Input: dimensioned drawing with shaded views. Units: mm. Origin: part minimum x, y, z. A direction names the side the tool comes from. Round coordinates to 2 decimals unless told otherwise and drop trailing zeros. Loops run counter-clockwise (first coordinate to the right, second up) from the corner with the lowest first, then second, coordinate; pieces in that order, holes last. Notation, with made-up numbers: (18.25, 78) - (59.25, 78) arc R20 ccw to (59.25, 104) - close; hole circle Ø8 at (80.5, 42). An arc over 180 degrees is marked (long way). One line per question, with ' | ' between items. Start each with the question number.
1. Cut plane A-A (x = 64.5). Return loops of the section in (y, z).
2. Pin query (flat end, axial travel): pin 1 (10 mm diameter, centred on x = 64, y = 84, fed in from +Z); pin 2 (5.5 mm diameter, centred on y = 80.5, z = 2.5, fed in from +X); pin 3 (5.5 mm diameter, centred on y = 34, z = 8.5, fed in from -X); pin 4 (4 mm diameter, centred on x = 131.5, z = 8.5, fed in from -Y). Return the tip coordinate at first contact, or that it passes through.
3. Cut plane C-C (z = 7.5). Return loops of the section in (x, y).
4. Cut plane B-B (y = 26.5). Return loops of the section in (x, z).
5. Cut plane D-D (x = 21.5). Return loops of the section in (y, z), then the cut area to 3 significant figures.
6. Ray query, line 1 (Y direction, x = 37, z = 3.5); line 2 (Z direction, x = 17, y = 57.5); line 3 (Y direction, x = 97, z = 8.5). Return the intervals inside material, ascending.
7. Access query for the marked faces 1, 2, 3 and 4. Directions: +Z, -Z, +X, -X, +Y, -Y. A direction counts if a zero-diameter tool reaches every point of the face in a straight line with its end or side. Return the directions, or none.
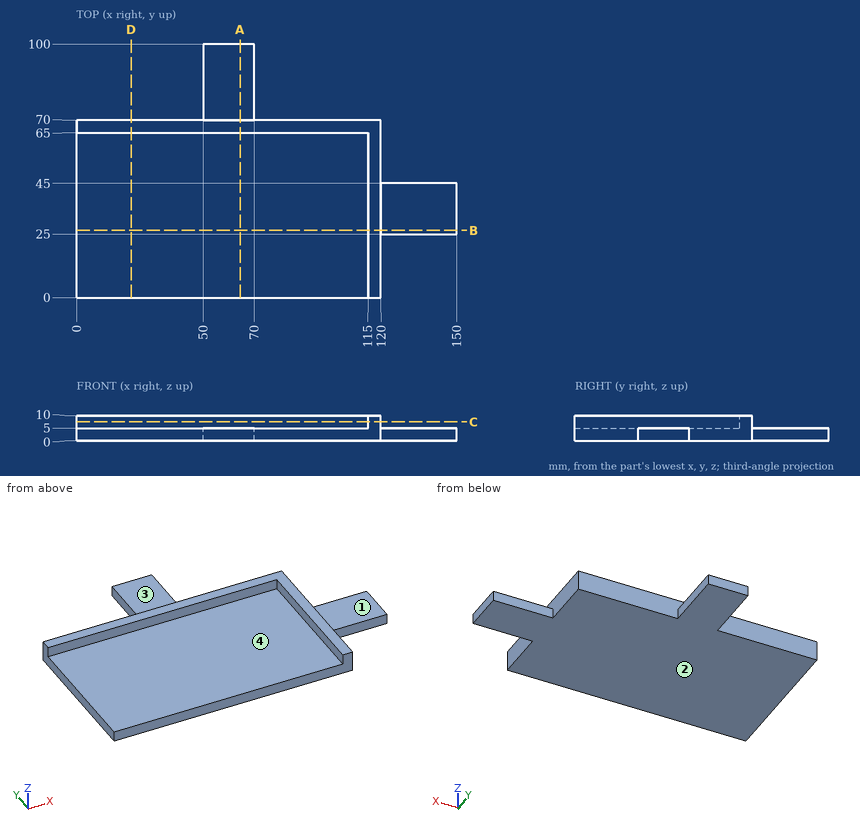
Answers follow:
1) outline: (0, 0) - (100, 0) - (100, 5) - (70, 5) - (70, 10) - (65, 10) - (65, 5) - (0, 5) - close
2) pin 1: stops at z = 5 | pin 2: stops at x = 70 | pin 3: stops at x = 115 | pin 4: passes through
3) outline: (0, 65) - (115, 65) - (115, 0) - (120, 0) - (120, 70) - (0, 70) - close
4) outline: (0, 0) - (150, 0) - (150, 5) - (120, 5) - (120, 10) - (115, 10) - (115, 5) - (0, 5) - close
5) outline: (0, 0) - (70, 0) - (70, 10) - (65, 10) - (65, 5) - (0, 5) - close | area: 375 mm2
6) line 1: y = 0 to 70 | line 2: z = 0 to 5 | line 3: y = 65 to 70
7) face 1: +Z, +X, +Y, -Y | face 2: -Z, +X, -X, +Y, -Y | face 3: +Z, +X, -X, +Y | face 4: +Z, -X, -Y
